CAD build for the part. Positions are in the model's coordinates, mm. A direction names the side the tool comes from. Coordinates: 2 decimals unless noted, no trailing zeros. Answer as a JSON object with one key per item and string values. Group by question number.
from build123d import *

# Parameters (mm, degrees)
SKETCH1_R           = 55.5625
BOSS_EXTRUDE1_DEPTH = 8.55
CHAMFER1_SIZE       = 3
SKETCH3_R           = 6.9
CUT_EXTRUDE1_DEPTH  = 4.4
SKETCH4_R           = 3.375
CUT_EXTRUDE2_DEPTH  = 4.15


with BuildPart() as part:
    # Sketch1 → Boss-Extrude1 (new body)
    with BuildSketch(Plane(origin=(0, 0, 0), x_dir=(0, 0, -1), z_dir=(1, 0, 0))):
        Circle(SKETCH1_R)
    extrude(amount=BOSS_EXTRUDE1_DEPTH)

    # Chamfer1
    chamfer1_edges = [part.edges().sort_by_distance(p)[0] for p in [
        (8.55, 0, 55.5625),
    ]]
    chamfer(chamfer1_edges, length=CHAMFER1_SIZE)

    # Sketch3 → Cut-Extrude1 (cut)
    with BuildSketch(Plane(origin=(8.55, 0, 0), x_dir=(0, 0, -1), z_dir=(1, 0, 0))):
        with Locations((0, 43.225)):
            Circle(SKETCH3_R)
        with Locations((0, -43.225)):
            Circle(SKETCH3_R)
    extrude(amount=-CUT_EXTRUDE1_DEPTH, mode=Mode.SUBTRACT)

    # Sketch4 → Cut-Extrude2 (cut)
    with BuildSketch(Plane(origin=(4.15, 0, 0), x_dir=(0, 0, -1), z_dir=(1, 0, 0))):
        with Locations((0, 43.225)):
            Circle(SKETCH4_R)
        with Locations((0, -43.225)):
            Circle(SKETCH4_R)
    extrude(amount=-CUT_EXTRUDE2_DEPTH, mode=Mode.SUBTRACT)


solid = part.part
Item 1: Band-saw the part on A-A, the plane z = 0. Count the separate pieces of the cut face and the enclosed holes in it, and give its area (3 significant figures).
Item 2: Pull direction Z, two halves, no side cores. Call faces 1 (the cylindrical face through (2.1, -39.88, 0.44)), 2 (the conical face through (8.404, -51.455, 11.426)), 3 (the flat face through (8.55, 1, 1)): +Z half, -Z half, draft (parallel to the pull), parting line (faces both ways), or undercut.
Item 3: Flat gauge pins, fed straight in: P1, Ø3, axis at x = 2.5, y = 23.5, coming from the -Z side; P2, Ø4, axis at x = 2, y = 32.5, coming from the -Z side; P3, Ø7, axis at y = 46, z = 1.5, coming from the +X side. Where does each tip first touch, or does it go through?
Item 4: Drill centre lines: L1, parallel to Y at x = 2.8, z = 0; L2, parallel to Y at x = 6.05, z = 0 (1 decimal); L3, parallel to Z at x = 4.5, y = -1.5. Where is each one in solid material? Low to high.
Item 5: 3-axis set-ups, long thin cutter, end or side, ignore diameter. For faces 4 (the flat face through (4.15, 40, 2)), 5 (the flat face through (0, 1, 1)): which of +Z, -Z, +X, -X, +Y, -Y reach the whole face in a straight line?
Reply:
{
 "1": {"separate pieces": "3", "enclosed holes": "0", "area": "764 mm²"},
 "2": {"face 1": "undercut", "face 2": "parting line", "face 3": "draft"},
 "3": {"P1": "z = -51.02", "P2": "z = -46.44", "P3": "x = 4.15"},
 "4": {"L1": "-55.56 to -46.6, -39.85 to 39.85, 46.6 to 55.56", "L2": "-55.1 to -50.1, -36.3 to 36.3, 50.1 to 55.1", "L3": "-55.54 to 55.54"},
 "5": {"face 4": "+X", "face 5": "+Z, -Z, -X, +Y, -Y"}
}
